Geometry: final body of the model. Coordinates: model frame, mm. Face numbers are marked on the shaded views. A direction names the side the tool comes from. Round coordinates to 2 decimals unless told otherwise and drop trailing zeros. Loops run counter-clockwise (first coordinate to the right, second up) from the corner with the lowest first, then second, coordinate; pieces in that order, holes last. Notation, with made-up numbers: M -5,-20.75 L 9,-20.75 A11 ccw 9,-3.75 Z; hole C -3,-28 d8. An arc over 180 degrees is marked long. Return JSON: item names as keys, results as strings.
from build123d import *

# Parameters (mm, degrees)
F0_R      = 6
F1_DEPTH  = 10
F2_W      = 52
F2_H      = 32
F3_DEPTH  = 650
F1_FACE_W = 50
F1_FACE_H = 10
F4_DEPTH  = 25
F6_DEPTH  = 40
F8_DEPTH  = 40


with BuildPart() as f1:
    # F0 (on Top) → F1 (new body)
    with BuildSketch(Plane.XY):
        with BuildLine():
            ThreePointArc((0, -25), (17.67767, -17.67767), (25, 0))
            ThreePointArc((25, 0), (17.67767, 17.67767), (0, 25))
            ThreePointArc((0, 25), (-25, 0), (0, -25))
        make_face()
        Circle(F0_R, mode=Mode.SUBTRACT)
        with BuildLine():
            ThreePointArc((0, -25), (-25, 0), (0, 25))
            Line((0, 25), (-50, 25))
            Line((-50, 25), (-50, -25))
            Line((-50, -25), (0, -25))
        make_face()
    extrude(amount=F1_DEPTH)



with BuildPart() as f3:
    # F2 (on face) → F3 (new body)
    with BuildSketch(Plane(origin=(-50, 0, 0), x_dir=(0, -1, 0), z_dir=(-1, 0, 0))):
        Polygon((30, 0), (0, 0), (-30, 0), (-30, -40), (30, -40), align=None)
        with Locations((0, -20)):
            Rectangle(F2_W, F2_H, mode=Mode.SUBTRACT)
    extrude(amount=F3_DEPTH)


with BuildPart() as f1_1:
    add(f1.part)

    add(f3.part)  # F4 merges F3
    # F1_face (on face) → F4 (join)
    with BuildSketch(Plane(origin=(-50, 0, 5), x_dir=(0, -1, 0), z_dir=(-1, 0, 0))):
        Rectangle(F1_FACE_W, F1_FACE_H)
    extrude(amount=F4_DEPTH)

    # F5 (on face) → F6 (cut)
    with BuildSketch(Plane.XY):
        with BuildLine():
            ThreePointArc((-369, 0), (-370.757359, 4.242641), (-375, 6))
            Line((-375, 6), (-375, 0))
            Line((-375, 0), (-369, 0))
        make_face()
        with BuildLine():
            ThreePointArc((-219, 0), (-225, 6), (-231, 0))
            ThreePointArc((-231, 0), (-225, -6), (-219, 0))
        make_face()
        with BuildLine():
            ThreePointArc((-269, 0), (-275, 6), (-281, 0))
            Line((-281, 0), (-275, 0))
            Line((-275, 0), (-269, 0))
        make_face()
        with BuildLine():
            Line((-275, 0), (-281, 0))
            ThreePointArc((-281, 0), (-275, -6), (-269, 0))
            Line((-269, 0), (-275, 0))
        make_face()
        with BuildLine():
            ThreePointArc((-319, 0), (-325, 6), (-331, 0))
            Line((-331, 0), (-325, 0))
            Line((-325, 0), (-319, 0))
        make_face()
        with BuildLine():
            Line((-325, 0), (-331, 0))
            ThreePointArc((-331, 0), (-325, -6), (-319, 0))
            Line((-319, 0), (-325, 0))
        make_face()
        with BuildLine():
            Line((-375, 0), (-375, 6))
            ThreePointArc((-375, 6), (-379.242641, -4.242641), (-369, 0))
            Line((-369, 0), (-375, 0))
        make_face()
    extrude(amount=-F6_DEPTH, mode=Mode.SUBTRACT)

    # F7 (on face) → F8 (cut)
    with BuildSketch(Plane.XY):
        with BuildLine():
            Line((-684, 30), (-700, 30))
            Line((-700, 30), (-700, 14))
            ThreePointArc((-700, 14), (-695.313708, 25.313708), (-684, 30))
        make_face()
        with BuildLine():
            ThreePointArc((-668, 14), (-672.686292, 25.313708), (-684, 30))
            ThreePointArc((-684, 30), (-695.313708, 25.313708), (-700, 14))
            ThreePointArc((-700, 14), (-684, -2), (-668, 14))
        make_face()
    extrude(amount=-F8_DEPTH, mode=Mode.SUBTRACT)


solid = f1_1.part
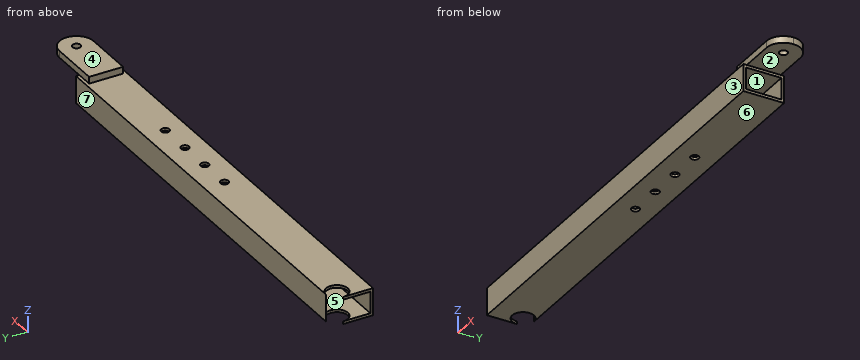
Q1. Pull-direction query (Z, two-part tool) for the marked faces 4, 5, 6 and 7; classes: pulls with the +Z half, pulls with the -Z half, needs draft (parallel to the pull), parting line crosses it, or undercut.
Determined:
{"face 4": "pulls with the +Z half", "face 5": "undercut", "face 6": "pulls with the -Z half", "face 7": "needs draft"}
Q2. Material intervals for L1, parallel to Y at x = -413, z = -14; L2, parallel to Z at x = -563.5, y = -22; L3, parallel to X at y = 0, z = -37, sorted ascending.
Determined:
{"L1": "y = -30 to -26, 26 to 30", "L2": "z = -40 to -36, -4 to 0", "L3": "x = -700 to -691.75, -676.25 to -381, -369 to -331, -319 to -281, -269 to -231, -219 to -50"}
Q3. Section query A-A (z = -29.5). Output: boundary loops of the cut face in (x, y).
Determined:
{"outline": "M -700,-30 L -50,-30 L -50,-26 L -700,-26 Z; M -684,30 A16 cw -673.42,26 L -50,26 L -50,30 Z"}
Q4. Pin query (flat end, axial travel): pin 1 (9.5 mm diameter, centred on x = -375, y = 0, fed in from +Z); pin 2 (5 mm diameter, centred on x = -512.5, y = -13, fed in from +Z); pin 3 (15 mm diameter, centred on x = -5, y = -2, fed in from -Z). Return the tip coordinate at first contact, or that it passes through.
Determined:
{"pin 1": "passes through", "pin 2": "stops at z = 0", "pin 3": "stops at z = 0"}
Q5. Reachability of the marked faces 1, 2 and 3 from +Z, -Z, +X, -X, +Y, -Y: full face, straight path, thin tool, end or side. Return the list, or none.
Determined:
{"face 1": "+X, -X", "face 2": "-Z, +X, +Y, -Y", "face 3": "+Z, -Z, +X, -X, -Y"}
Q6. Section query B-B (x = -225). Output: boundary loops of the cut face in (y, z), plus the area to 3 significant figures.
Determined:
{"outline": "M -30,-40 L -6,-40 L -6,-36 L -26,-36 L -26,-4 L -6,-4 L -6,0 L -30,0 Z; M 6,-40 L 30,-40 L 30,0 L 6,0 L 6,-4 L 26,-4 L 26,-36 L 6,-36 Z", "area": "640 mm^2"}
